Geometry check sheet. Reference: the model listing, model coordinates, mm. A direction names the side the tool comes from. Round coordinates to 2 decimals unless told otherwise and drop trailing zeros. Write each loop counter-clockwise with the first axis right and the second up, starting at its lowest first coordinate (ties: lowest second). Pieces come first, ordered by that corner, then holes.
Item 1: Scan lines: probe 1 along Z at (x, y) = (46, 62); probe 2 along X at (y, z) = (14.5, 4); probe 3 along Z at (x, y) = (-59.5, 58). Record each from-to range of solid material in increasing order.
Item 2: Access from +Z, -Z, +X, -X, +Y, -Y to the whole of each face (thin tool, end or side, straight path). Record for faces 4 (the face through (-15, 12.841, 184)), 5 (the face through (-4, 57, 118)), 6 (the face through (-36.48, 36.2, 186.11)), 7 (the face through (195, 27, 80)), 8 (the face through (160, 52, 0)).
Item 3: Cross-section at D-D (x = 175). Enter the section's corners in (y, z).
Item 4: Draft check along X on faces 1 (the face through (-5.502, 62.07, 128.613)), 2 (the face through (-36.48, 36.2, -186.11)), 3 (the face through (257.17, 27.34, -1.12)). Enter one of: pulls with the +X half, pulls with the -X half, needs draft (parallel to the pull), parting line crosses it, or undercut.
Item 5: Cross-section at A-A (z = 0). Enter the section's corners in (x, y), then the cut area to 3 significant figures.
Item 6: Cross-section at C-C (z = 121.5). Enter the section's corners in (x, y).
Item 7: Depth check by flat-ended pin: P1, Ø4, axis at x = -50.84, y = 11.69, coming from the +Z side; P2, Ø5, axis at x = -19, y = 26.5, coming from the +Z side; P3, Ø4, axis at x = 19.87, y = 11.69, coming from the -Z side; P4, Ø16, axis at x = 242.87, y = 15.46, coming from the -Z side. Enter the tip coordinate at first touch or a pass-through.
from build123d import *

# Parameters (mm, degrees)
SKETCH1_R                = 40
BOSS_EXTRUDE1_DEPTH      = 67
CUT_EXTRUDE1_DEPTH       = 10
BOSS_EXTRUDE2_DEPTH      = 80
CUT_EXTRUDE2_REACH       = 370.572
SKETCH4_R                = 10
FILLET1_R                = 15
CUT_EXTRUDE5_REACH       = 365.464
SKETCH6_W                = 20
SKETCH6_H                = 20
BOSS_EXTRUDE3_REACH      = 461.179
BOSS_EXTRUDE3_END_RADIUS = 172.5
SKETCH8_R                = 2.5
CUT_EXTRUDE6_DEPTH       = 40


with BuildPart() as part:
    # Sketch1 → Boss-Extrude1 (new body)
    with BuildSketch(Plane(origin=(0, 0, 0), x_dir=(1, 0, 0), z_dir=(0, 1, 0))):
        with BuildLine():
            Line((-152.827517156, 80), (-152.827517156, -80))
            ThreePointArc((-152.827517156, -80), (0, -172.5), (152.827517156, -80))
            Line((152.827517156, -80), (152.827517156, 80))
            ThreePointArc((152.827517156, 80), (0, 172.5), (-152.827517156, 80))
        make_face()
        with Locations(Location((0, 0, 0), (0, 0, 270))):
            Circle(SKETCH1_R, mode=Mode.SUBTRACT)
    extrude(amount=BOSS_EXTRUDE1_DEPTH)

    # Sketch2 → Cut-Extrude1 (cut)
    with BuildSketch(Plane(origin=(0, 67, 0), x_dir=(1, 0, 0), z_dir=(0, 1, 0))):
        with BuildLine():
            Line((-94.805792729, 77.709483627), (-94.766560633, 77.677326247))
            ThreePointArc((-94.766560633, 77.677326247), (-90.5175234, 76.33424343), (-86.514217379, 78.291723895))
            ThreePointArc((-86.514217379, 78.291723895), (0, 116.680348985), (86.514217379, 78.291723895))
            ThreePointArc((86.514217379, 78.291723895), (90.5175234, 76.33424343), (94.766560633, 77.677326247))
            Line((94.766560633, 77.677326247), (94.805792729, 77.709483627))
            ThreePointArc((94.805792729, 77.709483627), (96.985665668, 81.904305313), (95.451092594, 86.375710069))
            ThreePointArc((95.451092594, 86.375710069), (0, 128.731015561), (-95.451092594, 86.375710069))
            ThreePointArc((-95.451092594, 86.375710069), (-96.985665668, 81.904305313), (-94.805792729, 77.709483627))
        make_face()
        with BuildLine():
            Line((-94.805792729, -77.709483627), (-94.766560633, -77.677326247))
            ThreePointArc((-94.766560633, -77.677326247), (-90.5175234, -76.33424343), (-86.514217379, -78.291723895))
            ThreePointArc((-86.514217379, -78.291723895), (-6.261835306, -116.512202184), (77.624689613, -87.11321026))
            ThreePointArc((77.624689613, -87.11321026), (81.814735563, -85.59607355), (85.895347897, -87.386825304))
            Line((85.895347897, -87.386825304), (85.930907429, -87.423002288))
            ThreePointArc((85.930907429, -87.423002288), (87.648629228, -91.827296423), (85.643657226, -96.108471762))
            ThreePointArc((85.643657226, -96.108471762), (-6.90855337, -128.545502674), (-95.451092594, -86.375710069))
            ThreePointArc((-95.451092594, -86.375710069), (-96.985665668, -81.904305313), (-94.805792729, -77.709483627))
        make_face()
    extrude(amount=-CUT_EXTRUDE1_DEPTH, mode=Mode.SUBTRACT)

    # Sketch3 → Boss-Extrude2 (add, symmetric)
    with BuildSketch(Plane.XY):
        Polygon((152.827517156, 67), (260, 29.182962561), (260, 0), (152.827517156, 0), align=None)
    extrude(amount=BOSS_EXTRUDE2_DEPTH, both=True)

    # Sketch4 → Cut-Extrude2 (cut, up to next)
    with BuildSketch(Plane.XY.offset(80), mode=Mode.PRIVATE) as cut_extrude2_sk1:
        with Locations((197.867868221, 15.46479665)):
            Circle(SKETCH4_R)
    cut_extrude2_tool1 = extrude(cut_extrude2_sk1.sketch, amount=-CUT_EXTRUDE2_REACH, mode=Mode.PRIVATE) & part.part
    # Sketch4 → Cut-Extrude2 (cut, up to next)
    with BuildSketch(Plane.XY.offset(80), mode=Mode.PRIVATE) as cut_extrude2_sk2:
        with Locations((242.867868221, 15.46479665)):
            Circle(SKETCH4_R)
    cut_extrude2_tool2 = extrude(cut_extrude2_sk2.sketch, amount=-CUT_EXTRUDE2_REACH, mode=Mode.PRIVATE) & part.part
    add(cut_extrude2_tool1.solids().sort_by_distance((197.867868, 15.464797, 80))[0], mode=Mode.SUBTRACT)
    add(cut_extrude2_tool2.solids().sort_by_distance((242.867868, 15.464797, 80))[0], mode=Mode.SUBTRACT)

    # Fillet1
    fillet1_edges = [part.edges().sort_by_distance(p)[0] for p in [
        (260, 0, 0),
        (260, 29.182962561, 0),
    ]]
    fillet(fillet1_edges, radius=FILLET1_R)

    # Cut-Extrude5: up to this plane
    cut_extrude5_end = Plane(origin=(152.827517156, 67, 80), z_dir=(-0.3327532596919791, -0.9430139278740067, 0))
    # Sketch6 → Cut-Extrude5 (cut, up to the surface)
    with BuildSketch(Plane(origin=(160, 0, 0), x_dir=(0, 0, -1), z_dir=(1, 0, 0)), mode=Mode.PRIVATE) as cut_extrude5_sk1:
        with Locations((0, 52.234802616)):
            Rectangle(SKETCH6_W, SKETCH6_H)
    cut_extrude5_tool1 = split(extrude(cut_extrude5_sk1.sketch, amount=CUT_EXTRUDE5_REACH, mode=Mode.PRIVATE), bisect_by=cut_extrude5_end, keep=Keep.BOTH, mode=Mode.PRIVATE)
    add(cut_extrude5_tool1.solids().sort_by_distance((160, 52.234803, 0))[0], mode=Mode.SUBTRACT)

    # Boss-Extrude3: up to this cylinder (the profile starts outside it)
    boss_extrude3_end = Plane(origin=(0, 35.241624, 0), z_dir=(0, -1, 0)) * Cylinder(BOSS_EXTRUDE3_END_RADIUS, 1268.358, mode=Mode.PRIVATE)
    # Sketch7 → Boss-Extrude3 (add, up to the surface)
    with BuildSketch(Plane.XY.offset(200), mode=Mode.PRIVATE) as boss_extrude3_sk1:
        with BuildLine():
            Line((-18.820406998, 56.872330571), (-54.64630767, 14.938742986))
            ThreePointArc((-54.64630767, 14.938742986), (-55.385658765, 9.597966882), (-50.844780808, 6.690913939))
            Line((-50.844780808, 6.690913939), (19.866759041, 6.690913939))
            ThreePointArc((19.866759041, 6.690913939), (24.393824394, 9.568255396), (23.71052462, 14.888642223))
            Line((23.71052462, 14.888642223), (-11.175114557, 56.822229808))
            ThreePointArc((-11.175114557, 56.822229808), (-14.986115079, 58.624394168), (-18.820406998, 56.872330571))
        make_face()
        with BuildLine():
            Line((-18.798269892, 47.008349057), (-40.57573529, 21.054976432))
            ThreePointArc((-40.57573529, 21.054976432), (-41.277052009, 15.727947075), (-36.745513074, 12.841038384))
            Line((-36.745513074, 12.841038384), (6.809417721, 12.841038384))
            ThreePointArc((6.809417721, 12.841038384), (11.340956656, 15.727947075), (10.639639936, 21.054976432))
            Line((10.639639936, 21.054976432), (-11.137825461, 47.008349057))
            ThreePointArc((-11.137825461, 47.008349057), (-14.968047677, 48.794411009), (-18.798269892, 47.008349057))
        make_face(mode=Mode.SUBTRACT)
    boss_extrude3_tool1 = extrude(boss_extrude3_sk1.sketch, amount=-BOSS_EXTRUDE3_REACH, mode=Mode.PRIVATE) - boss_extrude3_end
    boss_extrude3 = boss_extrude3_tool1.solids().sort_by_distance((5.529884, 35.241624, 200))[0]
    add(boss_extrude3)

    # Sketch8 → Cut-Extrude6 (cut)
    with BuildSketch(Plane.XY.offset(200)):
        with Locations((-15.018880135, 53.624501524)):
            Circle(SKETCH8_R)
        with Locations((19.866759041, 11.690913939)):
            Circle(SKETCH8_R)
        with Locations((-50.844780808, 11.690913939)):
            Circle(SKETCH8_R)
    cut_extrude6 = extrude(amount=-CUT_EXTRUDE6_DEPTH, mode=Mode.SUBTRACT)

    # Mirror1: Boss-Extrude3, Cut-Extrude6 across plane
    add(boss_extrude3.mirror(Plane.XY))
    add(cut_extrude6.mirror(Plane.XY), mode=Mode.SUBTRACT)


solid = part.part
Resolved:
1. probe 1: z = -166.25 to -120.23, -107.23 to 107.23, 120.23 to 166.25
1. probe 2: x = -152.83 to -39.8, 39.8 to 187.91, 207.82 to 232.91, 252.82 to 259.99
1. probe 3: z = -161.91 to -114.16, -100.37 to 100.37, 114.16 to 161.91
2. face 4: +Z
2. face 5: +Y
2. face 6: +Z, -X, +Y
2. face 7: +Z, +X, +Y, -Y
2. face 8: +X
3. outline: (0, -80) - (59.18, -80) - (59.18, -10) - (42.23, -10) - (42.23, 10) - (59.18, 10) - (59.18, 80) - (0, 80) - close
4. face 1: undercut
4. face 2: pulls with the -X half
4. face 3: pulls with the +X half
5. outline: (-152.83, 0) - (-40, 0) - (-40, 67) - (-152.83, 67) - close; (40, 0) - (245, 0) arc R15 ccw to (260, 15) - (260, 18.57) arc R15 ccw to (249.99, 32.71) - (223.01, 42.23) - (160, 42.23) - (160, 62.23) - (166.33, 62.23) - (152.83, 67) - (40, 67) - close; hole circle Ø20 at (197.87, 15.46); hole circle Ø20 at (242.87, 15.46)
5. area: 18,900 mm2
6. outline: (-122.45, 0) - (122.45, 0) - (122.45, 67) - (42.54, 67) - (42.54, 57) - (-42.54, 57) - (-42.54, 67) - (-122.45, 67) - close
7. P1: stops at z = 160
7. P2: stops at z = 171.71
7. P3: stops at z = -160
7. P4: passes through
